The listing builds one solid part. Answer for the finished solid, in the listing's coordinates (mm). Face numbers are marked on the shaded views. A direction names the side the tool comes from. Give positions to 0.01 mm unless a question says otherwise; leave off trailing zeros. Loops run counter-clockwise (first coordinate to the right, second up) from the corner with the lowest first, then second, coordinate; pieces in that order, holes last. Notation, with made-up numbers: (25, 34.5) - (56, 34.5) arc R30 cw to (56, 56.5) - close; hole circle Ø8 at (-31, 79). An arc over 180 degrees is marked (long way). Answer as CSV lines item,"result". Start each with the question number.
1) A cutting plane is placed at A-A (x = -40). Determine the outline of the cut face in (y, z).
2) A cutting plane is placed at D-D (x = 18). Determine the outline of the cut face in (y, z).
3) Find the intervals of material crossed by line 1 along Y through (x, z) = (-17, 11); line 2 along X through (y, z) = (-1.5, 39); line 3 along X through (y, z) = (-49, 31.5), in increasing order.
4) For a pull along Y with two mould halves and no side action, classify the marked faces 1, 2, 3 and 4 as pulls with the +Y half, pulls with the -Y half, needs draft (parallel to the pull), parting line crosses it, or undercut.
5) A cutting plane is placed at C-C (y = 22). Determine the outline of the cut face in (x, z).
6) A flat-ended cylindrical pin translates along its axis: pin 1 (1.5 mm diameter, centred on x = 52, y = 36, fed in from -Z). Find the tip coordinate at first contact, or state that the pin passes through.
7) For the marked faces 5, 6, 7, 8 and 9, determine the directions among +Z, -Z, +X, -X, +Y, -Y from which every point of the face is accessible in a straight line to the end or side of a thin tool.
8) A cutting plane is placed at B-B (z = 31). Determine the outline of the cut face in (x, y).
```python
from build123d import *

# Parameters (mm, degrees)
SKETCH_1_W          = 140
SKETCH_1_H          = 130
SKETCH_1_R          = 36
SKETCH_1_W_2        = 20
SKETCH_1_H_2        = 20
EXTRUDE_1_DEPTH     = 50
SKETCH_2_R          = 39
CUT_EXTRUDE_1_DEPTH = 10
CUT_EXTRUDE_2_REACH = 132
SKETCH_3_W          = 40
SKETCH_3_H          = 50
SKETCH_4_R          = 3.75
SKETCH_4_W          = 38.75
SKETCH_4_H          = 7
CUT_EXTRUDE_3_DEPTH = 15
SKETCH_6_W          = 9.65
SKETCH_6_H          = 20.5
CUT_EXTRUDE_4_DEPTH = 51
SKETCH_7_W          = 29
SKETCH_7_H          = 20.5
CUT_EXTRUDE_5_DEPTH = 41


with BuildPart() as part:
    # 草圖1 → 填料-伸長1 (new body)
    with BuildSketch(Plane.XY):
        with Locations((8.56146046, -8.054151625)):
            Rectangle(SKETCH_1_W, SKETCH_1_H)
        with Locations((8.56146046, -8.054151625)):
            Circle(SKETCH_1_R, mode=Mode.SUBTRACT)
        with Locations((-45.43853954, -8.054151625)):
            Rectangle(SKETCH_1_W_2, SKETCH_1_H_2, mode=Mode.SUBTRACT)
        with Locations((62.56146046, -8.054151625)):
            Rectangle(SKETCH_1_W_2, SKETCH_1_H_2, mode=Mode.SUBTRACT)
    extrude(amount=EXTRUDE_1_DEPTH)

    # 草圖2 → 除料-伸長1 (cut)
    with BuildSketch(Plane(origin=(0, 0, 0), x_dir=(-1, 0, 0), z_dir=(0, 0, -1))):
        with Locations((-8.56146046, -8.054151625)):
            Circle(SKETCH_2_R)
    extrude(amount=-CUT_EXTRUDE_1_DEPTH, mode=Mode.SUBTRACT)

    # 草圖3 → 除料-伸長2 (cut, up to next)
    with BuildSketch(Plane.XZ.offset(73.054151625), mode=Mode.PRIVATE) as cut_extrude_2_sk1:
        with Locations((8.56146046, 25)):
            Rectangle(SKETCH_3_W, SKETCH_3_H)
    cut_extrude_2_tool1 = extrude(cut_extrude_2_sk1.sketch, amount=-CUT_EXTRUDE_2_REACH, mode=Mode.PRIVATE) & part.part
    add(cut_extrude_2_tool1.solids().sort_by_distance((8.56146, -73.054152, 25))[0], mode=Mode.SUBTRACT)

    # 草圖4 → 除料-伸長3 (cut)
    with BuildSketch(Plane(origin=(-11.43853954, 0, 0), x_dir=(0, 0, -1), z_dir=(1, 0, 0))):
        with Locations((-11.25, -48.054151625)):
            Circle(SKETCH_4_R)
        with Locations((-30.625, -48.304151625)):
            Rectangle(SKETCH_4_W, SKETCH_4_H)
    extrude(amount=-CUT_EXTRUDE_3_DEPTH, mode=Mode.SUBTRACT)

    # 草圖6 → 除料-伸長4 (cut, through all)
    with BuildSketch(Plane.XY.offset(50)):
        with Locations((33.38646046, -47.804151625)):
            Rectangle(SKETCH_6_W, SKETCH_6_H)
    extrude(amount=-CUT_EXTRUDE_4_DEPTH, mode=Mode.SUBTRACT)

    # 草圖7 → 除料-伸長5 (cut)
    with BuildSketch(Plane.XY.offset(50)):
        with Locations((52.71146046, -47.804151625)):
            Rectangle(SKETCH_7_W, SKETCH_7_H)
    extrude(amount=-CUT_EXTRUDE_5_DEPTH, mode=Mode.SUBTRACT)


solid = part.part
```
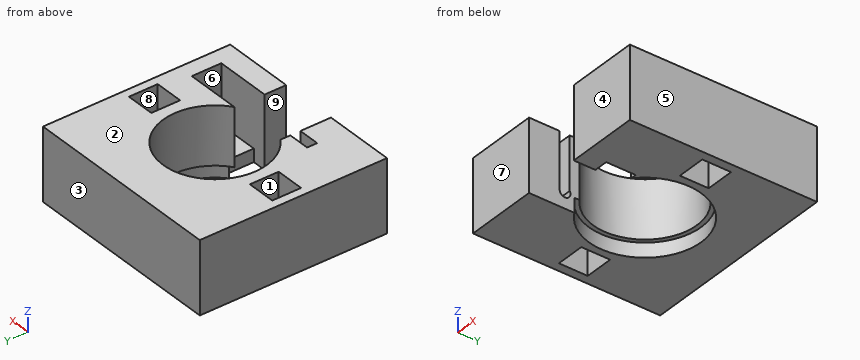
Ans:
1,outline,"(-73.05, 0) - (-18.05, 0) - (-18.05, 50) - (-73.05, 50) - close; (1.95, 0) - (56.95, 0) - (56.95, 50) - (1.95, 50) - close"
2,outline,"(26.69, 10) - (29.79, 10) - (29.79, 0) - (56.95, 0) - (56.95, 50) - (26.69, 50) - close"
3,line 1,"-73.05 to -51.8, -44.31 to -33.4, 17.3 to 56.95"
3,line 2,"-61.44 to -55.44, -35.44 to -26.84, 43.96 to 52.56, 72.56 to 78.56"
3,line 3,"-61.44 to -26.44, 67.21 to 78.56"
4,face 1,"undercut"
4,face 2,"needs draft"
4,face 3,"pulls with the +Y half"
4,face 4,"pulls with the -Y half"
5,outline,"(-61.44, 0) - (-16.29, 0) - (-16.29, 10) - (-11.26, 10) - (-11.26, 50) - (-61.44, 50) - close; (28.38, 10) - (33.42, 10) - (33.42, 0) - (78.56, 0) - (78.56, 50) - (28.38, 50) - close"
6,pin 1,"z = 0"
7,face 5,"+Z, -Z, +X, +Y, -Y"
7,face 6,"+Z"
7,face 7,"+Z, -Z, +X, -X, -Y"
7,face 8,"+Z, -Z"
7,face 9,"+Z, -Z, -Y"
8,outline,"(-61.44, -73.05) - (-11.44, -73.05) - (-11.44, -51.8) - (-26.44, -51.8) - (-26.44, -44.8) - (-11.44, -44.8) - (-11.44, -37.99) arc R36 cw (long way) to (29.2, -37.55) - (67.21, -37.55) - (67.21, -58.05) - (28.56, -58.05) - (28.56, -73.05) - (78.56, -73.05) - (78.56, 56.95) - (-61.44, 56.95) - close; hole (-55.44, -18.05) - (-35.44, -18.05) - (-35.44, 1.95) - (-55.44, 1.95) - close; hole (52.56, -18.05) - (72.56, -18.05) - (72.56, 1.95) - (52.56, 1.95) - close"
